For this review, take the finished solid that the model builds, in its own axes (mm). Give positions to 0.01 mm unless a question says otherwise; leave off trailing zeros. Write each loop counter-clockwise with the first axis right and the second up, starting at its lowest first coordinate (ties: lowest second). Pieces come first, ordered by that corner, then holes.
1) For P1, Ø1, axis at y = 2.5, z = 38, coming from the -X side, flat-tipped, find the tip position at first contact; note if it passes through.
2) We need section B-B on z = 0. Give the boundary of the cut face in (x, y), and give its area (3 significant figures).
3) Wall thickness on line 1 along X through (y, z) = (2.6, -42.5); line 2 along X through (y, z) = (1.6, -19); line 3 along X through (y, z) = (2.6, 0): over which ranges is each line inside the solid? List them lowest first.
4) Draft analysis for pull direction Z (two halves, no side actions). For faces 1 (the face through (45.65, 1.65, 46.27)), 2 (the face through (51, 3.35, 27)), 3 (the face through (42.16, 1.698, -44.403)), state which applies: pulls with the +Z half, pulls with the -Z half, needs draft (parallel to the pull), parting line crosses it, or undercut.
5) We need section A-A on x = 0. Give the boundary of the cut face in (y, z).
6) We need section C-C on y = 1.25. Give the boundary of the cut face in (x, z), and give its area (3 significant figures).
from build123d import *

# Parameters (mm, degrees)
SKETCH_1_R          = 65
SKETCH_1_R_2        = 57.15
EXTRUDE_1_DEPTH     = 3.35
SKETCH_2_W          = 162.249174321
SKETCH_2_H          = 152.83985105
SKETCH_2_W_2        = 124
SKETCH_2_H_2        = 124
CUT_EXTRUDE_1_DEPTH = 3.35
SKETCH_3_R          = 1.6
CUT_EXTRUDE_2_DEPTH = 3.35


with BuildPart() as part:
    # 草图1 → 凸台-拉伸1 (new body)
    with BuildSketch(Plane(origin=(0, 0, 0), x_dir=(1, 0, 0), z_dir=(0, 1, 0))):
        with Locations(Location((0, 0, 0), (0, 0, 270))):
            Circle(SKETCH_1_R)
        with Locations(Location((0, 0, 0), (0, 0, 270))):
            Circle(SKETCH_1_R_2, mode=Mode.SUBTRACT)
    extrude(amount=EXTRUDE_1_DEPTH)

    # 草图2 → 切除-拉伸1 (cut)
    with BuildSketch(Plane(origin=(0, 3.35, 0), x_dir=(1, 0, 0), z_dir=(0, 1, 0))):
        with Locations((0.017137102, 0)):
            Rectangle(SKETCH_2_W, SKETCH_2_H)
        Rectangle(SKETCH_2_W_2, SKETCH_2_H_2, mode=Mode.SUBTRACT)
    extrude(amount=-CUT_EXTRUDE_1_DEPTH, mode=Mode.SUBTRACT)

    # 草图3 → 切除-拉伸2 (cut)
    with BuildSketch(Plane(origin=(0, 3.35, 0), x_dir=(1, 0, 0), z_dir=(0, 1, 0))):
        with Locations(Location((43.133513652, -43.133513652, 0), (0, 0, 270))):
            Circle(SKETCH_3_R)
        with Locations(Location((-43.133513652, -43.133513652, 0), (0, 0, 270))):
            Circle(SKETCH_3_R)
        with Locations(Location((-43.133513652, 43.133513652, 0), (0, 0, 270))):
            Circle(SKETCH_3_R)
        with Locations(Location((43.133513652, 43.133513652, 0), (0, 0, 270))):
            Circle(SKETCH_3_R)
    extrude(amount=-CUT_EXTRUDE_2_DEPTH, mode=Mode.SUBTRACT)


solid = part.part
Results list:
1. P1: stops at x = -53.09
2. outline: (-62, 0) - (-57.15, 0) - (-57.15, 3.35) - (-62, 3.35) - close; (57.15, 0) - (62, 0) - (62, 3.35) - (57.15, 3.35) - close
2. area: 32.5 mm2
3. line 1: x = -49.18 to -44.6, -41.66 to -38.21, 38.21 to 41.66, 44.6 to 49.18
3. line 2: x = -62 to -53.9, 53.9 to 62
3. line 3: x = -62 to -57.15, 57.15 to 62
4. face 1: pulls with the +Z half
4. face 2: needs draft
4. face 3: undercut
5. outline: (0, -62) - (3.35, -62) - (3.35, -57.15) - (0, -57.15) - close; (0, 57.15) - (3.35, 57.15) - (3.35, 62) - (0, 62) - close
6. outline: (-62, -19.52) arc R65 ccw to (-19.52, -62) - (19.52, -62) arc R65 ccw to (62, -19.52) - (62, 19.52) arc R65 ccw to (19.52, 62) - (-19.52, 62) arc R65 ccw to (-62, 19.52) - close; hole circle Ø114.3 at (0, 0); hole circle Ø3.2 at (-43.13, -43.13); hole circle Ø3.2 at (-43.13, 43.13); hole circle Ø3.2 at (43.13, -43.13); hole circle Ø3.2 at (43.13, 43.13)
6. area: 2,670 mm2
